Geometry: final body of the model. Coordinates: model frame, mm. A direction names the side the tool comes from. Coordinates: 2 decimals unless noted, no trailing zeros. Order: outer loops, then holes, each group sorted by start corner. A loop starts at its lowest first (then second) coordinate and runs counter-clockwise, first axis right, second up. Notation, with made-up numbers: M 73,65 L 105,65 A17 cw 105,71 Z; hole C 30,-16 d3. An arc over 180 degrees is marked long. One line per question, with ' | ' between items.
from build123d import *

# Parameters (mm, degrees)
BOSS_EXTRUDE1_DEPTH = 2.1536931
CUT_EXTRUDE1_REACH  = 56.318
SKETCH3_W           = 2.1536931
SKETCH3_H           = 7
SKETCH4_W           = 2.1536931
SKETCH4_H           = 8.5489795
BOSS_EXTRUDE2_DEPTH = 3.9


with BuildPart() as part:
    # Sketch1 → Boss-Extrude1 (new body)
    with BuildSketch(Plane.XY):
        Polygon((28, 0), (-28, 0), (-28, 15.5489795), (-24, 15.5489795), (-24, 8.5489795), (24, 8.5489795), (24, 15.5489795), (28, 15.5489795), align=None)
    extrude(amount=BOSS_EXTRUDE1_DEPTH)

    # Sketch3 → Cut-Extrude1 (cut, up to next)
    with BuildSketch(Plane.ZY.offset(-24), mode=Mode.PRIVATE) as cut_extrude1_sk1:
        with Locations((1.07684655, 12.0489795)):
            Rectangle(SKETCH3_W, SKETCH3_H)
    cut_extrude1_tool1 = extrude(cut_extrude1_sk1.sketch, amount=-CUT_EXTRUDE1_REACH, mode=Mode.PRIVATE) & part.part
    add(cut_extrude1_tool1.solids().sort_by_distance((24, 12.048979, 1.076847))[0], mode=Mode.SUBTRACT)

    # Sketch4 → Boss-Extrude2 (add)
    with BuildSketch(Plane(origin=(28, 0, 0), x_dir=(0, 0, -1), z_dir=(1, 0, 0))):
        with Locations((-1.07684655, 4.27448975)):
            Rectangle(SKETCH4_W, SKETCH4_H)
    extrude(amount=BOSS_EXTRUDE2_DEPTH)


solid = part.part
1. Material intervals for line 1 (Y direction, x = -9, z = 1.85); line 2 (X direction, y = 9.75, z = 1.7), sorted ascending. Write a range as [from, to].
Response values:
line 1: y = [0, 8.55] | line 2: x = [-28, -24]
2. Section C-C, the plane x = 4. Output: boundary loops of the cut face in (y, z), and give its area (3 significant figures).
Response values:
outline: M 0,0 L 8.55,0 L 8.55,2.15 L 0,2.15 Z | area: 18.4 mm^2
3. Section A-A, the plane z = 1.65. Output: boundary loops of the cut face in (x, y), and give its area (3 significant figures).
Response values:
outline: M -28,0 L 31.9,0 L 31.9,8.55 L -24,8.55 L -24,15.55 L -28,15.55 Z | area: 540 mm^2
4. Section B-B, the plane y = 14.25. Output: boundary loops of the cut face in (x, z), and give its area (3 significant figures).
Response values:
outline: M -28,0 L -24,0 L -24,2.15 L -28,2.15 Z | area: 8.61 mm^2
5. Pin query (flat end, axial travel): P1, Ø6, axis at x = 6, y = 9.5, coming from the -Z side; P2, Ø1, axis at x = 9, y = 9.5, coming from the +Z side. Return the tip coordinate at first contact, or that it passes through.
Response values:
P1: stops at z = 0 | P2: passes through
6. Access query for faces 1 (the face through (-24, 12, 1)), 2 (the face through (2, 4, 0)). Directions: +Z, -Z, +X, -X, +Y, -Y. A direction counts if a zero-diameter tool reaches every point of the face in a straight line with its end or side. Return the directions, or none.
Response values:
face 1: +Z, -Z, +X, +Y | face 2: -Z, +X, -X, +Y, -Y
